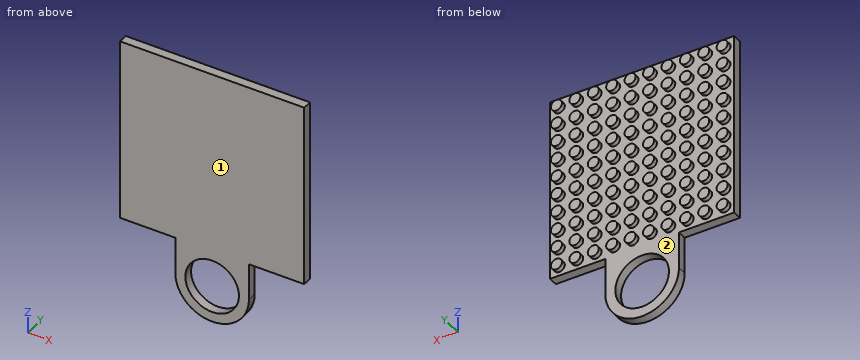
from build123d import *

# Parameters (mm, degrees)
SKETCH1_W               = 10
SKETCH1_H               = 10
PLATE_DEPTH             = 0.5
SKETCH2_R               = 0.3
ROD_DEPTH               = 0.25
LPATTERN1_COUNT         = 10
LPATTERN1_PITCH         = 1
LPATTERN1_COUNT_DIR2    = 10
LPATTERN1_PITCH_DIR2    = 1
BOSS_EXTRUDE3_DEPTH     = 0.5
SKETCH5_R               = 1.455938962
CUT_EXTRUDE1_DEPTH      = 0.5
CUT_EXTRUDE1_DEPTH_BACK = 1.5


with BuildPart() as part:
    # Sketch1 → Plate (new body)
    with BuildSketch(Plane(origin=(0, 0, 0), x_dir=(1, 0, 0), z_dir=(0, 1, 0))):
        Rectangle(SKETCH1_W, SKETCH1_H)
    extrude(amount=PLATE_DEPTH)

    # Sketch2 → Rod (add)
    with BuildSketch(Plane(origin=(0, 0.5, 0), x_dir=(1, 0, 0), z_dir=(0, 1, 0))):
        with Locations((-4.5, -4.5)):
            Circle(SKETCH2_R)
    rod = extrude(amount=ROD_DEPTH)

    # LPattern1: Rod 10 × 10
    with Locations(*[(i * LPATTERN1_PITCH, 0, -j * LPATTERN1_PITCH_DIR2) for i in range(LPATTERN1_COUNT) for j in range(LPATTERN1_COUNT_DIR2) if (i, j) != (0, 0)]):
        add(rod)

    # Sketch4 → Boss-Extrude3 (add)
    with BuildSketch(Plane(origin=(0, 0, 0), x_dir=(1, 0, 0), z_dir=(0, 1, 0))):
        with BuildLine():
            Line((-2, 7), (-2, 5))
            Line((-2, 5), (2, 5))
            Line((2, 5), (2, 7))
            ThreePointArc((2, 7), (0, 9), (-2, 7))
        make_face()
    extrude(amount=BOSS_EXTRUDE3_DEPTH)

    # Sketch5 → Cut-Extrude1 (cut, two sides)
    with BuildSketch(Plane(origin=(0, 0.5, 0), x_dir=(1, 0, 0), z_dir=(0, 1, 0))) as cut_extrude1_sk:
        with Locations((0, 7)):
            Circle(SKETCH5_R)
    extrude(amount=CUT_EXTRUDE1_DEPTH, mode=Mode.SUBTRACT)
    extrude(cut_extrude1_sk.sketch, amount=-CUT_EXTRUDE1_DEPTH_BACK, mode=Mode.SUBTRACT)


solid = part.part
Design review of the part built by this model. Coordinates are the model's own, in mm. Face numbers are marked on the shaded views. Round coordinates to 2 decimals unless told otherwise and drop trailing zeros. Loops run counter-clockwise (first coordinate to the right, second up) from the corner with the lowest first, then second, coordinate; pieces in that order, holes last. Notation, with made-up numbers: (89, 9) - (102, 9) arc R22 cw to (102, 36) - close; hole circle Ø7 at (73.25, -33). An arc over 180 degrees is marked (long way). One line per item, written item: value. Start each with the question number.
1) Consider section B-B on z = 4. Give the boundary of the cut face in (x, y), then the cut area to 3 significant figures.
2) To check wall thickness, follow L1, parallel to Z at x = 0, y = 0.2; L2, parallel to X at y = 0.2, z = -7; L3, parallel to Z at x = -2.25, y = 0.35. State the ranges of each line that lie inside material, in increasing order. Write a range as from..to.
3) Consider section A-A on x = 0. Give the boundary of the cut face in (y, z), then the cut area to 3 significant figures.
4) Draft analysis for pull direction X (two halves, no side actions). For the marked faces 1 and 2, state which applies: +X half, -X half, draft (parallel to the pull), parting line (faces both ways), or undercut.
Reported:
1. outline: (-5, 0) - (5, 0) - (5, 0.5) - (-5, 0.5) - close
1. area: 5.00 mm^2
2. L1: z = -9..-8.46, -5.54..5
2. L2: x = -2..-1.46, 1.46..2
2. L3: z = -5..5
3. outline: (0, -9) - (0.5, -9) - (0.5, -8.46) - (0, -8.46) - close; (0, -5.54) - (0.5, -5.54) - (0.5, 5) - (0, 5) - close
3. area: 5.54 mm^2
4. face 1: draft
4. face 2: undercut
